Verification items for the finished model (mm, model axes). A direction names the side the tool comes from. Round coordinates to 2 decimals unless told otherwise and drop trailing zeros. Write each loop counter-clockwise with the first axis right and the second up, starting at its lowest first coordinate (ties: lowest second). Pieces come first, ordered by that corner, then holes. Notation, with made-up numbers: (11.5, -39.75) -> (33.5, -39.75) arc R13 cw to (33.5, -31.75) -> close; hole circle Ø6 at (12, 49). An arc over 180 degrees is marked (long way). Use CSV: the item, a comma, the result in double quotes.
```python
from build123d import *

# Parameters (mm, degrees)
SZKIC4_R                   = 4
WYTNIJ_WYCI_GNI_CIE1_DEPTH = 10
SZKIC5_R                   = 13
WYTNIJ_WYCI_GNI_CIE2_DEPTH = 10


with BuildPart() as part:
    # Szkic1 → Obrót1 (revolve)
    with BuildSketch(Plane.XY):
        Polygon((-90, -36.5), (-70, -36.5), (-70, -47), (-48, -47), (-48, -138), (52, -138), (52, -58), (63, -58), (63, -49.5), (73, -49.5), (78, -44.5), (78, -38.5), (90, -38.5), (90, 0), (-90, 0), align=None)
    revolve(axis=Axis((90, 0, 0), (-1, 0, 0)))

    # Szkic4 → Wytnij-wyciągnięcie1 (cut)
    with BuildSketch(Plane(origin=(90, 0, 0), x_dir=(0, 0, -1), z_dir=(1, 0, 0))):
        with Locations((16, 27.712812921)):
            Circle(SZKIC4_R)
        with Locations((32, 0)):
            Circle(SZKIC4_R)
        with Locations((16, -27.712812921)):
            Circle(SZKIC4_R)
        with Locations((-16, -27.712812921)):
            Circle(SZKIC4_R)
        with Locations((-32, 0)):
            Circle(SZKIC4_R)
        with Locations((-16, 27.712812921)):
            Circle(SZKIC4_R)
    extrude(amount=-WYTNIJ_WYCI_GNI_CIE1_DEPTH, mode=Mode.SUBTRACT)

    # Szkic5 → Wytnij-wyciągnięcie2 (cut)
    with BuildSketch(Plane(origin=(90, 0, 0), x_dir=(0, 0, -1), z_dir=(1, 0, 0))):
        Circle(SZKIC5_R)
    extrude(amount=-WYTNIJ_WYCI_GNI_CIE2_DEPTH, mode=Mode.SUBTRACT)


solid = part.part
```
Q1. Access from +Z, -Z, +X, -X, +Y, -Y to the whole of each face (thin tool, end or side, straight path). Record for faces 4 (the flat face through (80, 28, -16)), 5 (the flat face through (-48, -2, -59)), 6 (the flat face through (90, 1, -17)).
Filled in:
face 4,"+X"
face 5,"-X"
face 6,"+Z, -Z, +X, +Y, -Y"
Q2. Mould release check, pull along Z, two halves, no side actions. Record for faces 1 (the flat face through (80, 28, 16)), 2 (the cylindrical face through (-58.85, -44.83, 14.12)), 3 (the flat face through (78, 20, 33.2)): released by +Z, released by -Z, zero draft, split by the parting line, or undercut.
Filled in:
face 1,"undercut"
face 2,"split by the parting line"
face 3,"zero draft"
Q3. Go/stop test with flat-tipped pins: P1, Ø6, axis at x = 1, z = -22, coming from the +Y side; P2, Ø4, axis at y = -27, z = -15.5, coming from the +X side; P3, Ø5, axis at x = 7.5, z = 77, coming from the +Y side. Record where each tip stops, or that it passes through.
Filled in:
P1,"y = 136.69"
P2,"x = 80"
P3,"y = 116.16"
Q4. Section check B-B (x = 43). Record the cut outline in (y, z).
Filled in:
outline,"circle Ø276 at (0, 0)"
Q5. Material ranges on L1, parallel to Y at x = 87, z = -16; L2, parallel to X at y = 55.5, z = -52; L3, parallel to X at y = 25, z = -46, recorded low to high.
Filled in:
L1,"-35.02 to -31.71, -23.71 to 23.71, 31.71 to 35.02"
L2,"-48 to 52"
L3,"-48 to 63"
Q6. Section check C-C (y = -82.5). Record the cut outline in (x, z).
Filled in:
outline,"(-48, -110.62) -> (52, -110.62) -> (52, 110.62) -> (-48, 110.62) -> close"
Q7. Section check D-D (z = 78). Record the cut outline in (x, y), plus the area to 3 significant figures.
Filled in:
outline,"(-48, -113.84) -> (52, -113.84) -> (52, 113.84) -> (-48, 113.84) -> close"
area,"22,800 mm²"
